```python
from build123d import *

# Parameters (mm, degrees)
F1_DEPTH      = 14
F2_R          = 2.75
F3_DEPTH      = 6
F4_R          = 1
F5_R          = 2
F6_DEPTH      = 10
F6_DEPTH_BACK = 9
F7_R          = 0.5


with BuildPart() as f1:
    # F0 (on Front) → F1 (new body)
    with BuildSketch(Plane.XZ):
        with BuildLine():
            Line((-9, 6), (-21, 6))
            Line((-21, 6), (-21, 0))
            Line((-21, 0), (21, 0))
            Line((21, 0), (21, 6))
            Line((21, 6), (9, 6))
            Line((9, 6), (9, 32.8))
            Line((9, 32.8), (1, 32.8))
            Line((1, 32.8), (1, 23.8729833462))
            ThreePointArc((1, 23.8729833462), (0, 16), (-1, 23.8729833462))
            Line((-1, 23.8729833462), (-1, 32.8))
            Line((-1, 32.8), (-9, 32.8))
            Line((-9, 32.8), (-9, 6))
        make_face()
    extrude(amount=F1_DEPTH)

    # F2 (on Top) → F3 (cut)
    with BuildSketch(Plane.XY):
        with Locations((16, -7)):
            Circle(F2_R)
        with Locations((-16, -7)):
            Circle(F2_R)
    extrude(amount=F3_DEPTH, mode=Mode.SUBTRACT)

    # F4
    f4_edges = [f1.edges().sort_by_distance(p)[0] for p in [
        (-21, -7, 6),
        (-15, 0, 6),
        (-15, -14, 6),
        (15, -14, 6),
        (21, -7, 6),
        (15, 0, 6),
        (-9, -7, 32.8),
        (9, -7, 32.8),
        (5, 0, 32.8),
        (-5, 0, 32.8),
        (-5, -14, 32.8),
        (5, -14, 32.8),
    ]]
    fillet(f4_edges, radius=F4_R)

    # F5 (on Right) → F6 (cut, two sides)
    with BuildSketch(Plane.YZ) as f6_sk:
        with Locations((-7, 28)):
            Circle(F5_R)
    extrude(amount=-F6_DEPTH, mode=Mode.SUBTRACT)
    extrude(f6_sk.sketch, amount=F6_DEPTH_BACK, mode=Mode.SUBTRACT)

    # F7
    f7_edges = [f1.edges().sort_by_distance(p)[0] for p in [
        (1, -9, 28),
        (-9, -9, 28),
        (-1, -9, 28),
    ]]
    fillet(f7_edges, radius=F7_R)


solid = f1.part
```
Part model, mm, in its own coordinate system. A direction names the side the tool comes from. Round coordinates to 2 decimals unless told otherwise and drop trailing zeros. Loops run counter-clockwise (first coordinate to the right, second up) from the corner with the lowest first, then second, coordinate; pieces in that order, holes last.
1. Slice it at C-C (z = 3.5). Give the cut face in (x, y).
Solutions:
outline: (-21, -14) - (21, -14) - (21, 0) - (-21, 0) - close; hole circle Ø5.5 at (-16, -7); hole circle Ø5.5 at (16, -7)
2. 3-axis set-ups, long thin cutter, end or side, ignore diameter. For faces 4 (the face through (13, -6, 6)), 5 (the face through (-15.084, -13.699, 5.715)), 6 (the face through (-13, -7, 6)): which of +Z, -Z, +X, -X, +Y, -Y reach the whole face in a straight line?
Solutions:
face 4: +Z, +X, +Y, -Y
face 5: +Z, -X, -Y
face 6: +Z, -X, +Y, -Y
3. Drill centre lines: line 1 along X through (y, z) = (-0.25, 29.5); line 2 along X through (y, z) = (-5, 3); line 3 along Z through (x, y) = (-4.25, -7). Where is each one in solid material? Low to high.
Solutions:
line 1: x = -9 to -1, 1 to 9
line 2: x = -21 to -17.89, -14.11 to 14.11, 17.89 to 21
line 3: z = 0 to 26, 30 to 32.8
4. Two-plate mould, pull along Z, no slides. Class faces 1 (the face through (-2, -14, 12)), 2 (the face through (5, -7, 26)), 3 (the face through (-20.699, -7.098, 5.715)): pulls with the +Z half, pulls with the -Z half, needs draft (parallel to the pull), parting line crosses it, or undercut.
Solutions:
face 1: needs draft
face 2: undercut
face 3: pulls with the +Z half
5. Slice it at D-D (y = -7). Count the separate pieces of the cut face and the enclosed holes in it, and give its area (3 significant figures).
Solutions:
separate pieces: 5
enclosed holes: 0
area: 535 mm2
6. Flat gauge pins, fed straight in: pin 1 (1 mm diameter, centred on x = 12, y = -6.5, fed in from +Z); pin 2 (7 mm diameter, centred on y = -8, z = 15.5, fed in from +X); pin 3 (3 mm diameter, centred on y = -7, z = 28, fed in from +X) (3 decimals); pin 4 (2.5 mm diameter, centred on y = -4, z = 28.5, fed in from -X). Where does each tip first touch, or does it go through?
Solutions:
pin 1: stops at z = 6
pin 2: stops at x = 9
pin 3: passes through
pin 4: stops at x = -9
7. Slice it at A-A (x = -16). Give the cut face in (y, z), and give its area (3 significant figures).
Solutions:
outline: (-14, 0) - (-9.75, 0) - (-9.75, 6) - (-13, 6) arc R1 ccw to (-14, 5) - close; (-4.25, 0) - (0, 0) - (0, 5) arc R1 ccw to (-1, 6) - (-4.25, 6) - close
area: 50.6 mm2
8. Slice it at B-B (x = 6). Give the cut face in (y, z), and give its area (3 significant figures).
Solutions:
outline: (-14, 0) - (0, 0) - (0, 31.8) arc R1 ccw to (-1, 32.8) - (-13, 32.8) arc R1 ccw to (-14, 31.8) - close; hole circle Ø4 at (-7, 28)
area: 446 mm2
